Could you check a few things on this model? Use its own coordinates, in mm. Face numbers are marked on the shaded views. A direction names the side the tool comes from. Round coordinates to 2 decimals unless told otherwise and drop trailing zeros. Loops run counter-clockwise (first coordinate to the right, second up) from the corner with the lowest first, then second, coordinate; pieces in that order, holes last. Notation, with made-up numbers: (85.5, -25.5) -> (132.5, -25.5) arc R24 ccw to (132.5, -10.5) -> close; hole circle Ø2 at (72, 25). An arc over 180 degrees is marked (long way). One line per item, written item: value.
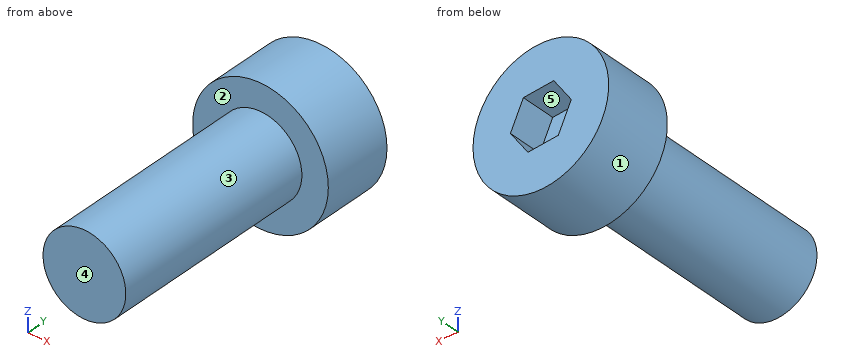
Autodesk Inventor part; units mm, degrees
ref_plane "YZ Plane" through (0, 0, 0) normal (1, 0, 0) x (0, 1, 0)
ref_plane "XZ Plane" through (0, 0, 0) normal (0, 1, 0) x (-1, 0, 0)
ref_plane "XY Plane" through (0, 0, 0) normal (0, 0, 1) x (1, 0, 0)
sketch "Sketch1" plane through (0, 0, 0) normal (0, 1, 0) x (-1, 0, 0)
  circle A0 centre (0, 0) radius 1.175
  dimension "d0" = 2.35
extrude "Extrusion1" add sketch "Sketch1" along normal blind 6
sketch "Sketch2" plane through (0, 6, 0) normal (0, 1, 0) x (1, 0, 0)
  circle A0 centre (0, 0) radius 1.175
  circle A1 centre (0, 0) radius 1.925
  dimension "d3" = 3.85
extrude "Extrusion2" add sketch "Sketch2" along normal blind 2 contours A0 | A1
sketch "Sketch3" plane through (0, 8, 0) normal (0, 1, 0) x (1, 0, 0)
  line L0 (-0.4961, 0.7099) -> (0.3667, 0.7845)
  line L1 (0.3667, 0.7845) -> (0.8628, 0.0747)
  line L2 (0.8628, 0.0747) -> (0.4961, -0.7099)
  line L3 (0.4961, -0.7099) -> (-0.3667, -0.7845)
  line L4 (-0.3667, -0.7845) -> (-0.8628, -0.0747)
  line L5 (-0.8628, -0.0747) -> (-0.4961, 0.7099)
  point P0 (0, 0)
  point P1 (0, 0)
  dimension "d6" = 1.5
extrude "Extrusion3" cut sketch "Sketch3" against normal blind 1
equation "\"d0\" = M2_A"
equation "\"d3\" = M2_B"
properties part number "M2_SCREW_8MM"
Item 1: If we section it at C-C on y = 2: List the corners of the cut face in (x, z) for me (3 decimals).
Output:
outline: circle Ø2.35 at (0, 0)
Item 2: For the marked faces 1 and 2, which set-ups out of +Z, -Z, +X, -X, +Y, -Y let a thin tool reach every point of the face, with its end or its side?
Output:
face 1: +Y, -Y
face 2: -Y
Item 3: If we mould it in two halves opening along X, with no side actions, what happens to the marked faces 3, 4 and 5? For each: released by +X, released by -X, zero draft, split by the parting line, or undercut.
Output:
face 3: split by the parting line
face 4: zero draft
face 5: undercut
Item 4: I need wall thicknesses on line 1 (Y direction, x = 0.45, z = 1.65); line 2 (Y direction, x = -0.15, z = 0.45); line 3 (Z direction, x = 0.4, y = 1.5). Which ranges of each line are inside material? Lowest first, please. Write a range as from..to.
Output:
line 1: y = 6..8
line 2: y = 0..7
line 3: z = -1.1..1.1
Item 5: If we section it at B-B on x = 0: List the corners of the cut face in (y, z) for me (3 decimals), plus the area to 3 significant figures.
Output:
outline: (0, -1.175) -> (6, -1.175) -> (6, -1.925) -> (8, -1.925) -> (8, -0.753) -> (7, -0.753) -> (7, 0.753) -> (8, 0.753) -> (8, 1.925) -> (6, 1.925) -> (6, 1.175) -> (0, 1.175) -> close
area: 20.3 mm²
Item 6: If we section it at A-A on z = 0.2: List the corners of the cut face in (x, y) for me.
Output:
outline: (-1.91, 6) -> (-1.16, 6) -> (-1.16, 0) -> (1.16, 0) -> (1.16, 6) -> (1.91, 6) -> (1.91, 8) -> (0.73, 8) -> (0.73, 7) -> (-0.78, 7) -> (-0.78, 8) -> (-1.91, 8) -> close
Item 7: Will these pins go through, and if not, where does the flat tip stop? pin 1 Ø2 at (y, z) = (4.5, 0) entering from -X (3 decimals); pin 2 Ø1 at (x, y) = (-0.5, 3) entering from +Z (3 decimals); pin 3 Ø1.5 at (x, z) = (-0.5, -1.5) entering from -Y.
Output:
pin 1: stops at x = -1.175
pin 2: stops at z = 1.175
pin 3: stops at y = 0
Item 8: If we section it at D-D on z = 1.35: List the corners of the cut face in (x, y) for me, plus the area to 3 significant figures.
Output:
outline: (-1.37, 6) -> (1.37, 6) -> (1.37, 8) -> (-1.37, 8) -> close
area: 5.49 mm²
